The drawing under review shows one solid part. Ordinate dimensions are in mm from its lowest x, y, z. Coordinates: 2 decimals unless noted, no trailing zeros. Write each loop counter-clockwise with the first axis right and the second up, starting at its lowest first coordinate (ties: lowest second). Pieces come first, ordered by that corner, then holes. Notation, with made-up numbers: (37.25, 38.5) -> (90.25, 38.5) arc R12 ccw to (90.25, 56.5) -> close; hole circle Ø3 at (-23.5, 16). An arc over 180 degrees is marked (long way). One line per item, written item: value. Start each with the question number.
1) For probe 1 along X at (y, z) = (87, 306); probe 2 along Z at (x, y) = (452, 122.5), list the stretches that pass through material, from the lowest coordinate up. Write a range as from..to.
2) Add section A-A (x = 101.6). State the section outline as (y, z) points, and give its area (3 significant figures).
3) Mouldability with a two-part tool opening along Y and no side actions: class the marked faces 1, 2 and 3 as released by +Y, released by -Y, zero draft, split by the parting line, or undercut.
4) For pin 1 Ø1.5 at (x, y) = (129.5, 42) entering from +Z, flat-tipped, find the tip position at first contact; note if it passes through.
5) Add section D-D (y = 63). State the section outline as (x, z) points.
6) Add section B-B (y = 215). State the section outline as (x, z) points, and give its area (3 significant figures).
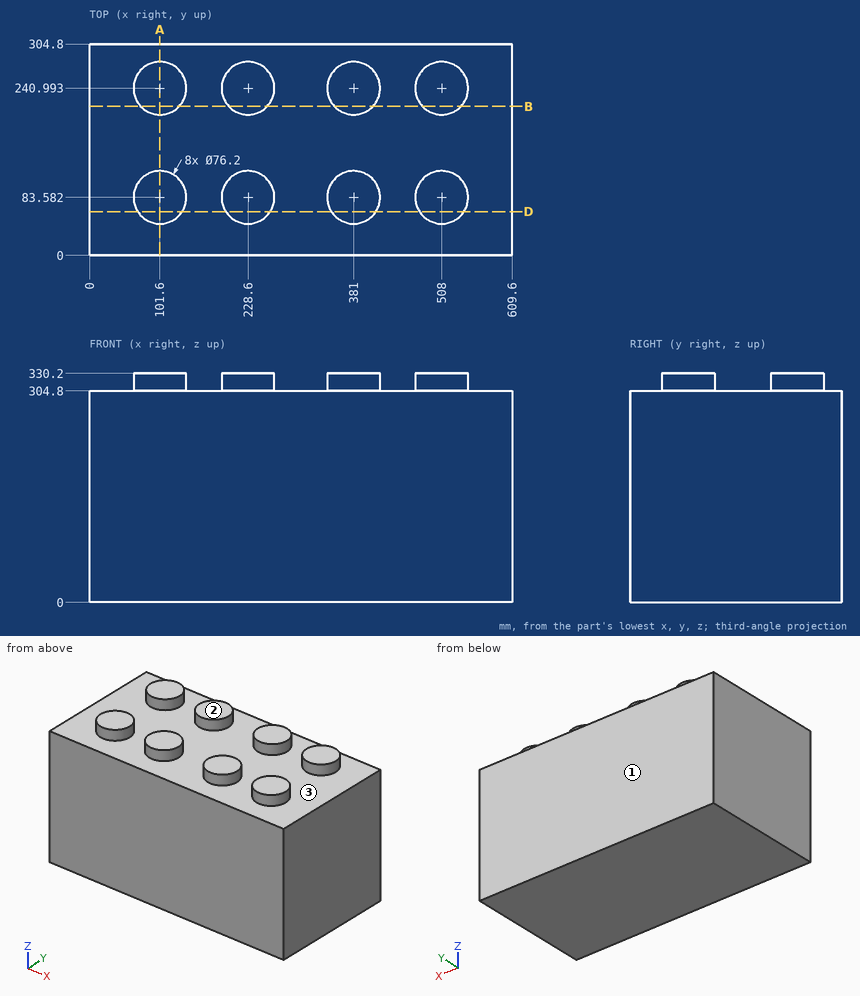
Numbers:
1. probe 1: 63.65..139.55, 190.65..266.55, 343.05..418.95, 470.05..545.95
1. probe 2: 0..304.8
2. outline: (0, 0) -> (304.8, 0) -> (304.8, 304.8) -> (279.09, 304.8) -> (279.09, 330.2) -> (202.89, 330.2) -> (202.89, 304.8) -> (121.68, 304.8) -> (121.68, 330.2) -> (45.48, 330.2) -> (45.48, 304.8) -> (0, 304.8) -> close
2. area: 96,800 mm²
3. face 1: released by +Y
3. face 2: zero draft
3. face 3: undercut
4. pin 1: z = 304.8
5. outline: (0, 0) -> (609.6, 0) -> (609.6, 304.8) -> (540.06, 304.8) -> (540.06, 330.2) -> (475.94, 330.2) -> (475.94, 304.8) -> (413.06, 304.8) -> (413.06, 330.2) -> (348.94, 330.2) -> (348.94, 304.8) -> (260.66, 304.8) -> (260.66, 330.2) -> (196.54, 330.2) -> (196.54, 304.8) -> (133.66, 304.8) -> (133.66, 330.2) -> (69.54, 330.2) -> (69.54, 304.8) -> (0, 304.8) -> close
6. outline: (0, 0) -> (609.6, 0) -> (609.6, 304.8) -> (535.86, 304.8) -> (535.86, 330.2) -> (480.14, 330.2) -> (480.14, 304.8) -> (408.86, 304.8) -> (408.86, 330.2) -> (353.14, 330.2) -> (353.14, 304.8) -> (256.46, 304.8) -> (256.46, 330.2) -> (200.74, 330.2) -> (200.74, 304.8) -> (129.46, 304.8) -> (129.46, 330.2) -> (73.74, 330.2) -> (73.74, 304.8) -> (0, 304.8) -> close
6. area: 191,000 mm²
